Autodesk Inventor part; units mm, degrees
ref_plane "YZ Plane" through (0, 0, 0) normal (1, 0, 0) x (0, 1, 0)
ref_plane "XZ Plane" through (0, 0, 0) normal (0, 1, 0) x (-1, 0, 0)
ref_plane "XY Plane" through (0, 0, 0) normal (0, 0, 1) x (1, 0, 0)
sketch "Sketch1" plane through (0, 0, 0) normal (0, 0, 1) x (1, 0, 0)
  line L0 (0, 0) -> (100, 0)
  line L1 (100, 0) -> (100, -75)
  line L2 (100, -75) -> (75, -118.3013)
  line L3 (75, -118.3013) -> (-12.5, -118.3013)
  line L4 (-12.5, -118.3013) -> (-12.5, -50)
  arc A0 (0, 0) -> (-12.5, -50) centre (77.4072, -45.9143) ccw
  dimension "d0" = 100
  dimension "d1" = 75
  dimension "d2" = 50
  dimension "d3" = 150
  dimension "d5" = 50
  dimension "d6" = 12.5
  dimension "d7" = 90
extrude "Extrusion1" add sketch "Sketch1" along normal blind 50
sketch "Sketch2" plane through (0, 0, 0) normal (0, 0, -1) x (-1, 0, 0)
  line L0 (0, 0) -> (-100, 0)
  line L1 (-100, 0) -> (-100, -75)
  line L2 (-100, -75) -> (-75, -118.3013)
  line L3 (-75, -118.3013) -> (12.5, -118.3013)
  line L4 (12.5, -118.3013) -> (12.5, -50)
  arc A0 (12.5, -50) -> (0, 0) centre (-77.4072, -45.9143) ccw
  line L5 (-95, -73.6603) -> (-95, -5)
  line L6 (-95, -5) -> (-2.902, -5)
  arc A1 (7.5, -49.8848) -> (-2.902, -5) centre (-77.4072, -45.9143) ccw
  line L7 (7.5, -49.8848) -> (7.5, -113.3013)
  line L8 (7.5, -113.3013) -> (-72.1132, -113.3013)
  line L9 (-72.1132, -113.3013) -> (-95, -73.6603)
  dimension "d10" = 5
extrude "Extrusion2" cut sketch "Sketch2" against normal blind 45 contours L5 L6 A1 L7 L8 L9
sketch "Sketch3" plane through (0, 0, 0) normal (0, 0, -1) x (-1, 0, 0)
  line L0 (7.5, -113.3013) -> (-72.1132, -113.3013)
  line L1 (12.5, -118.3013) -> (-75, -118.3013)
  line L2 (7.5, -113.3013) -> (-60, -113.3013)
  line L3 (-60, -113.3013) -> (-60, -118.3013)
  line L4 (-60, -118.3013) -> (7.5, -118.3013)
  line L5 (7.5, -118.3013) -> (7.5, -113.3013)
  point P0 (0, 0)
  dimension "d13" = 15
extrude "Extrusion3" cut sketch "Sketch3" against normal blind 45
sketch "Sketch4" plane through (0, 0, 0) normal (0, 1, 0) x (1, 0, 0)
  circle A0 centre (50, 0) radius 10
  line L0 (0, 0) -> (100, 0)
  dimension "d16" = 20
extrude "Extrusion4" cut sketch "Sketch4" against normal through all
sketch "Sketch5" plane through (0, 0, 50) normal (0, 1, 0) x (1, 0, 0)
  arc A0 (40, 50) -> (60, 50) centre (50, 50) ccw
  circle A1 centre (50, 50) radius 30 construction
  circle A2 centre (50, 20) radius 2.5
  circle A3 centre (75.9808, 35) radius 2.5
  circle A4 centre (75.9808, 65) radius 2.5
  circle A5 centre (50, 80) radius 2.5
  circle A6 centre (24.0192, 65) radius 2.5
  circle A7 centre (24.0192, 35) radius 2.5
  point P0 (0, 50)
  dimension "d19" = 60
  dimension "d20" = 5
  dimension "d23" = 360
extrude "Extrusion5" cut sketch "Sketch5" against normal blind 5 contours A2 | A3 | A7
sketch "Sketch6" plane through (0, 0, 50) normal (0, 0, 1) x (1, 0, 0)
  circle A0 centre (25, -25) radius 7.5
  point P0 (0, 0)
  dimension "d27" = 15
  dimension "d28" = 25
  dimension "d29" = 25
extrude "Extrusion6" cut sketch "Sketch6" against normal blind 5
sketch "Sketch7" plane through (-12.5, -118.3013, 50) normal (0, -1, 0) x (1, 0, 0)
  line L0 (87.5, 0) -> (112.5, 0)
  line L1 (87.5, 0) -> (32.5, 0)
  line L2 (32.5, 0) -> (32.5, -15)
  line L3 (32.5, -15) -> (87.5, -15)
  line L4 (87.5, -15) -> (87.5, 0)
  line L5 (0, -50) -> (0, 0)
  point P0 (12.5, -50)
  dimension "d32" = 15
  dimension "d33" = 32.5
extrude "Extrusion7" add sketch "Sketch7" against normal blind 5
sketch "Sketch9" plane through (0, 0, 0) normal (0, 0, -1) x (-1, 0, 0)
  circle A0 centre (-65, -40) radius 6
  circle A1 centre (-22.5, -58.3013) radius 6
  line L0 (-100, 0) -> (-100, -75)
  line L1 (-60, 0) -> (-100, 0)
  line L2 (12.5, -118.3013) -> (12.5, -50)
  line L3 (7.5, -118.3013) -> (-20, -118.3013)
  point P0 (0, 0)
  point P1 (-57.5, 0)
  dimension "d39" = 12
  dimension "d40" = 12
  dimension "d41" = 35
  dimension "d42" = 40
  dimension "d43" = 35
  dimension "d44" = 60
extrude "Extrusion9" cut sketch "Sketch9" against normal through all
sketch "Sketch10" plane through (0, 0, 45) normal (0, 0, -1) x (-1, 0, 0)
  circle A0 centre (-65, -40) radius 6
  circle A1 centre (-22.5, -58.3013) radius 6
  circle A2 centre (-22.5, -58.3013) radius 10
  circle A3 centre (-65, -40) radius 10
  point P0 (0, 0)
  dimension "d47" = 20
  dimension "d48" = 20
extrude "Extrusion10" add sketch "Sketch10" along normal blind 45
sketch "Sketch11" plane through (65, -40, 0) normal (0, 0, -1) x (-1, 0, 0)
  circle A0 centre (0, 0) radius 10
  circle A1 centre (42.5, -18.3013) radius 10
  circle A2 centre (42.5, -18.3013) radius 6
  circle A3 centre (0, 0) radius 6
  circle A4 centre (42.5, -18.3013) radius 2.5
  circle A5 centre (0, 0) radius 6
  circle A6 centre (0, 0) radius 2.5
  point P0 (65, 40)
  dimension "d51" = 5
  dimension "d52" = 5
extrude "Extrusion11" add sketch "Sketch11" against normal blind 10 contours A2 | A3
properties part number "FA002" material "ABS Plastic"
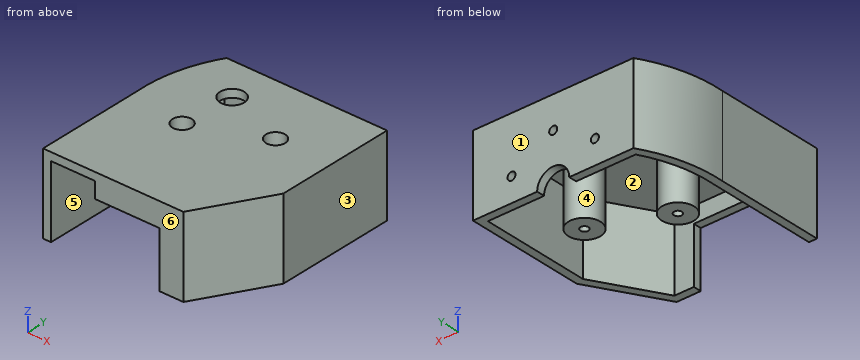
Input: part model. Units: mm. Frame: model coordinates. Face numbers are marked on the shaded views. A direction names the side the tool comes from. Give positions to 0.01 mm unless a question says otherwise; leave off trailing zeros. Order: outer loops, then holes, each group sorted by start corner. A loop starts at its lowest first (then second) coordinate and runs counter-clockwise, first axis right, second up. Notation, with made-up numbers: M -18.75,-33.75 L 27.25,-33.75 A24 cw 27.25,-13.75 Z; hole C 63,21 d7. An arc over 180 degrees is marked long. One line per question, with ' | ' between items. Start each with the question number.
1. Access query for the marked faces 4, 5 and 6. Directions: +Z, -Z, +X, -X, +Y, -Y. A direction counts if a zero-diameter tool reaches every point of the face in a straight line with its end or side. Return the directions, or none.
2. Pull-direction query (Y, two-part tool) for the marked faces 1, 2 and 3; classes: released by +Y, released by -Y, zero draft, split by the parting line, or undercut.
3. Section query B-B (y = -20.5). Return the cut outline in (x, z), and give its area (3 significant figures).
4. First-contact query: pin 1 Ø2.5 at (x, y) = (40.5, -116) entering from -Z; pin 2 Ø19.5 at (x, y) = (25, -25) entering from +Z; pin 3 Ø2 at (x, y) = (82.5, -23) entering from -Z; pin 4 Ø3.5 at (x, y) = (66, -40) entering from +Z. Flat tips, straight axial feed; report the tip coordinate or a pass-through.
5. Material intervals for probe 1 along Y at (x, z) = (65, 19.5); probe 2 along X at (y, z) = (-1, 15); probe 3 along X at (y, z) = (-2, 15), sorted ascending. Write a range as [from, to].
6. Section query C-C (x = 65). Return the cut outline in (y, z).
7. Section query D-D (z = 39). Return the cut outline in (x, y).
8. Section query A-A (z = 15). Return the cut outline in (x, y), and give its area (3 significant figures).
Here are the results:
1) face 4: -Z | face 5: -Z, -Y | face 6: +Z, -Z, +X, -X, -Y
2) face 1: released by +Y | face 2: undercut | face 3: zero draft
3) outline: M -8.93,0 L -3.7,0 L -3.7,45 L 19,45 L 19,50 L -8.93,50 Z; M 31,45 L 95,45 L 95,0 L 100,0 L 100,50 L 31,50 Z | area: 945 mm²
4) pin 1: z = 35 | pin 2: z = 50 | pin 3: z = 45 | pin 4: z = 10
5) probe 1: [-118.3, -113.3], [-50, -46], [-34, -30], [-5, 0] | probe 2: [-0.58, 21.52], [26.52, 73.48], [78.48, 100] | probe 3: [-1.15, 21.52], [26.52, 73.48], [78.48, 100]
6) outline: M -118.3,0 L -113.3,0 L -113.3,45 L -50,45 L -50,0 L -42.5,0 L -42.5,10 L -46,10 L -46,50 L -118.3,50 Z; M -37.5,0 L -30,0 L -30,45 L -5,45 L -5,0 L 0,0 L 0,50 L -34,50 L -34,10 L -37.5,10 Z
7) outline: M -12.5,-118.3 L -7.5,-118.3 L -7.5,-49.88 A85 cw 2.9,-5 L 95,-5 L 95,-73.66 L 72.11,-113.3 L 20,-113.3 L 20,-118.3 L 75,-118.3 L 100,-75 L 100,0 L 0,0 A90 ccw -12.5,-50 Z; C 22.5,-58.3 d20; C 65,-40 d20; hole C 22.5,-58.3 d12; hole C 65,-40 d12
8) outline: M -12.5,-118.3 L -7.5,-118.3 L -7.5,-49.88 A85 cw 2.9,-5 L 21.52,-5 L 21.52,0 L 0,0 A90 ccw -12.5,-50 Z; C 22.5,-58.3 d20; M 26.52,-5 L 73.48,-5 L 73.48,0 L 26.52,0 Z; C 65,-40 d20; M 60,-118.3 L 75,-118.3 L 100,-75 L 100,0 L 78.48,0 L 78.48,-5 L 95,-5 L 95,-73.66 L 72.11,-113.3 L 60,-113.3 Z; hole C 22.5,-58.3 d12; hole C 65,-40 d12 | area: 2,090 mm²
